Build history of the part. All positions in model axes, mm. Face numbers are marked on the shaded views. A direction names the side the tool comes from. Round coordinates to 2 decimals unless told otherwise and drop trailing zeros. Write each loop counter-clockwise with the first axis right and the second up, starting at its lowest first coordinate (ties: lowest second). Pieces come first, ordered by that corner, then holes. Notation, with made-up numbers: M 35,-10 L 54,-10 A18 cw 54,18 Z; hole C 18,-12 d1. An arc over 180 degrees is marked long. Write item = value, one per line.
from build123d import *

# Parameters (mm, degrees)
BOSS_EXTRUDE4_DEPTH = 12
SKETCH3_4_R         = 5
SKETCH3_4_R_2       = 2.5
BOSS_EXTRUDE5_DEPTH = 3
BOSS_EXTRUDE6_START = -9
SKETCH3_5_R         = 5
SKETCH3_5_R_2       = 2.5
BOSS_EXTRUDE6_DEPTH = 3
BOSS_EXTRUDE7_START = -12
SKETCH2_R           = 10
BOSS_EXTRUDE7_DEPTH = 15
BOSS_EXTRUDE8_START = 15
SKETCH5_R           = 15
BOSS_EXTRUDE8_DEPTH = 15


with BuildPart() as part:
    # Sketch3 → Boss-Extrude4 (new body)
    with BuildSketch(Plane.XY):
        with BuildLine():
            ThreePointArc((15, 0), (14.999214481, 0.153508816), (14.996858006, 0.307001554))
            ThreePointArc((14.996858006, 0.307001554), (-10.606601718, 10.606601718), (-0.307001554, -14.996858006))
            ThreePointArc((-0.307001554, -14.996858006), (10.497499147, -10.714593397), (15, 0))
        make_face()
        with BuildLine():
            ThreePointArc((4.1, 0), (-2.074849392, -3.536240942), (-2, 3.579106034))
            Line((-2, 3.579106034), (-2, 5.1))
            Line((-2, 5.1), (2, 5.1))
            Line((2, 5.1), (2, 3.579106034))
            ThreePointArc((2, 3.579106034), (3.536240942, 2.074849392), (4.1, 0))
        make_face(mode=Mode.SUBTRACT)
    extrude(amount=-BOSS_EXTRUDE4_DEPTH)

    # Sketch3<4> → Boss-Extrude5 (add)
    # profile 1 of 2: a face of its own
    with BuildSketch(Plane.XY):
        with BuildLine():
            ThreePointArc((15.918131612, -22.562761855), (14.495689014, -14.495689014), (22.562761855, -15.918131612))
            Line((22.562761855, -15.918131612), (14.996858006, 0.307001554))
            ThreePointArc((14.996858006, 0.307001554), (14.999214481, 0.153508816), (15, 0))
            ThreePointArc((15, 0), (10.497499147, -10.714593397), (-0.307001554, -14.996858006))
            Line((-0.307001554, -14.996858006), (15.918131612, -22.562761855))
        make_face()
    # profile 2 of 2: a face of its own
    with BuildSketch(Plane.XY):
        with Locations((18.03122292, -18.03122292)):
            Circle(SKETCH3_4_R)
        with Locations((18.03122292, -18.03122292)):
            Circle(SKETCH3_4_R_2, mode=Mode.SUBTRACT)
    extrude(amount=-BOSS_EXTRUDE5_DEPTH)

    # Sketch3<5> → Boss-Extrude6 (add)
    # profile 1 of 2: a face of its own
    with BuildSketch(Plane.XY.offset(BOSS_EXTRUDE6_START)):
        with BuildLine():
            ThreePointArc((15.918131612, -22.562761855), (14.495689014, -14.495689014), (22.562761855, -15.918131612))
            Line((22.562761855, -15.918131612), (14.996858006, 0.307001554))
            ThreePointArc((14.996858006, 0.307001554), (14.999214481, 0.153508816), (15, 0))
            ThreePointArc((15, 0), (10.497499147, -10.714593397), (-0.307001554, -14.996858006))
            Line((-0.307001554, -14.996858006), (15.918131612, -22.562761855))
        make_face()
    # profile 2 of 2: a face of its own
    with BuildSketch(Plane.XY.offset(BOSS_EXTRUDE6_START)):
        with Locations((18.03122292, -18.03122292)):
            Circle(SKETCH3_5_R)
        with Locations((18.03122292, -18.03122292)):
            Circle(SKETCH3_5_R_2, mode=Mode.SUBTRACT)
    extrude(amount=-BOSS_EXTRUDE6_DEPTH)

    # Sketch2 → Boss-Extrude7 (add)
    with BuildSketch(Plane.XY.offset(BOSS_EXTRUDE7_START)):
        Circle(SKETCH2_R)
        with BuildLine():
            ThreePointArc((4.1, 0), (-2.074849392, -3.536240942), (-2, 3.579106034))
            Line((-2, 3.579106034), (-2, 5.1))
            Line((-2, 5.1), (2, 5.1))
            Line((2, 5.1), (2, 3.579106034))
            ThreePointArc((2, 3.579106034), (3.536240942, 2.074849392), (4.1, 0))
        make_face(mode=Mode.SUBTRACT)
    extrude(amount=-BOSS_EXTRUDE7_DEPTH)

    # Sketch5 → Boss-Extrude8 (add)
    with BuildSketch(Plane.XY.offset(BOSS_EXTRUDE8_START)):
        Circle(SKETCH5_R)
        with BuildLine():
            Line((-3, 9.224424101), (-3, 11.8))
            Line((-3, 11.8), (3, 11.8))
            Line((3, 11.8), (3, 9.224424101))
            ThreePointArc((3, 9.224424101), (7.848248212, 5.70043858), (9.7, 0))
            ThreePointArc((9.7, 0), (-5.70043858, -7.848248212), (-3, 9.224424101))
        make_face(mode=Mode.SUBTRACT)
    extrude(amount=-BOSS_EXTRUDE8_DEPTH)


solid = part.part
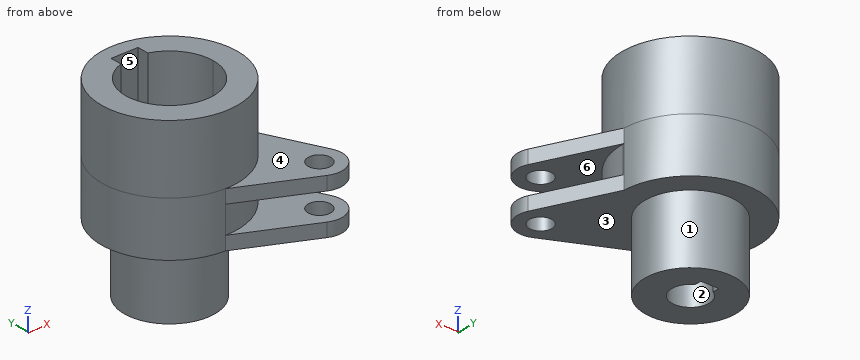
1. Probe probe 1 along Z at (x, y) = (14, -14); probe 2 along Y at (x, z) = (0, 6); probe 3 along X at (y, z) = (0, 11). List the from-to ranges inside material, lowest first.
Responses:
probe_1 = -12 to -9, -3 to 0
probe_2 = -15 to -9.7, 11.8 to 15
probe_3 = -15 to -9.7, 9.7 to 15
2. Band-saw the part on D-D (x = 13). List the corners of the cut face in (y, z).
Responses:
outline = M -21.2,-12 L 7.48,-12 L 7.48,15 L -7.48,15 L -7.48,0 L -21.2,0 L -21.2,-3 L -7.48,-3 L -7.48,-9 L -21.2,-9 Z
3. Mould opens along Y. For the marked faces 1, 2 and 3 say: pulls with the +Y half, pulls with the -Y half, needs draft (parallel to the pull), parting line crosses it, or undercut.
Responses:
face_1 = parting line crosses it
face_2 = undercut
face_3 = needs draft
4. Band-saw the part on B-B (x = 17). List the corners of the cut face in (y, z).
Responses:
outline = M -22.92,-12 L -20.31,-12 L -20.31,-9 L -22.92,-9 Z; M -22.92,-3 L -20.31,-3 L -20.31,0 L -22.92,0 Z; M -15.75,-12 L -3.99,-12 L -3.99,-9 L -15.75,-9 Z; M -15.75,-3 L -3.99,-3 L -3.99,0 L -15.75,0 Z
5. Band-saw the part on A-A (z = 4). List the corners of the cut face in (x, y).
Responses:
outline = C 0,0 d30; hole M -3,9.22 A9.7 ccw long 3,9.22 L 3,11.8 L -3,11.8 Z
6. Band-saw the part on C-C (y = 1). List the corners of the cut face in (x, z), plus the area to 3 significant figures.
Responses:
outline = M -14.97,-12 L -9.95,-12 L -9.95,-27 L -3.98,-27 L -3.98,0 L -9.65,0 L -9.65,15 L -14.97,15 Z; M 3.98,-27 L 9.95,-27 L 9.95,-12 L 14.97,-12 L 14.97,15 L 9.65,15 L 9.65,0 L 3.98,0 Z
area = 603 mm²
7. Tool access for the marked faces 4, 5 and 6: list every direction of +Z, -Z, +X, -X, +Y, -Y with a clear straight run to the whole face (end or side of a thin tool).
Responses:
face_4 = +Z, +X, -Y
face_5 = +Z
face_6 = +X, -Y
8. Flat gauge pins, fed straight in: pin 1 (0.8 mm diameter, centred on y = 10.5, z = 11, fed in from -X); pin 2 (1.2 mm diameter, centred on y = 4.5, z = -8, fed in from +X); pin 3 (5 mm diameter, centred on x = 0, y = 0, fed in from -Z); pin 4 (19 mm diameter, centred on x = 8.5, y = -8.5, fed in from -Z). Where does each tip first touch, or does it go through?
Responses:
pin_1 = -11.09
pin_2 = 14.48
pin_3 = through
pin_4 = -27
